Build history of the part. All positions in model axes, mm. A direction names the side the tool comes from. Give positions to 0.01 mm unless a question says otherwise; leave off trailing zeros. Order: outer loops, then holes, each group sorted by start corner. A loop starts at its lowest first (then second) coordinate and runs counter-clockwise, first axis right, second up. Notation, with made-up numbers: (-10, 42) - (12, 42) arc R13 ccw to (12, 58) - close; hole circle Ø1 at (37, 29.5). An arc over 180 degrees is marked (long way). Use a Markdown table: item, result.
Autodesk Inventor part; units mm, degrees
ref_plane "YZ Plane" through (0, 0, 0) normal (1, 0, 0) x (0, 1, 0)
ref_plane "XZ Plane" through (0, 0, 0) normal (0, 1, 0) x (-1, 0, 0)
ref_plane "XY Plane" through (0, 0, 0) normal (0, 0, 1) x (1, 0, 0)
sketch "Boceto1" plane through (0, 0, 0) normal (0, 1, 0) x (-1, 0, 0)
  circle A0 centre (0, 0) radius 10.2
  circle A1 centre (0, 0) radius 12.2
  dimension "d0" = 20.4
  dimension "d1" = 2
extrude "Extrusión1" add sketch "Boceto1" along normal blind 2
sketch "Boceto2" plane through (0, 2, 0) normal (0, 1, 0) x (1, 0, 0)
  circle A0 centre (0, 0) radius 12.2
  circle A1 centre (0, 0) radius 10.2
  circle A2 centre (0, 0) radius 2.25
  dimension "d4" = 4.5
extrude "Extrusión2" add sketch "Boceto2" along normal blind 4 contours A0 | A1
sketch "Boceto3" plane through (0, 6, 0) normal (0, 1, 0) x (1, 0, 0)
  circle A0 centre (0, 0) radius 5
  dimension "d7" = 10
extrude "Extrusión3" cut sketch "Boceto3" against normal blind 2
properties part number "springsupport"
1) Wall check: line 1 (X direction, y = 5.4, z = 0); line 2 (Z direction, x = 0, y = 3.25). Give the ranges that are in metal, low to high. Write a range as from..to.
Computed:
| item | result |
|---|---|
| line 1 | x = -12.2..-5, 5..12.2 |
| line 2 | z = -12.2..-2.25, 2.25..12.2 |
2) Slice it at B-B (z = -1). Write the cut outline in (x, y), and give its area (3 significant figures).
Computed:
| item | result |
|---|---|
| outline | (-12.16, 0) - (-10.15, 0) - (-10.15, 2) - (-2.02, 2) - (-2.02, 4) - (-4.9, 4) - (-4.9, 6) - (-12.16, 6) - close; (2.02, 2) - (10.15, 2) - (10.15, 0) - (12.16, 0) - (12.16, 6) - (4.9, 6) - (4.9, 4) - (2.02, 4) - close |
| area | 77.6 mm² |
3) Tool access for faces 1 (the flat face through (-0.1, 2, -2.4)), 2 (the flat face through (2.2, 4, 1)), 3 (the flat face through (3, 0, -10)): list every direction of +Z, -Z, +X, -X, +Y, -Y with a clear straight run to the whole face (end or side of a thin tool).
Computed:
| item | result |
|---|---|
| face 1 | -Y |
| face 2 | +Y |
| face 3 | +Z, -Z, +X, -X, -Y |
4) Pin check, flat tips, straight feed: P1, Ø1, axis at x = -10, y = 3, coming from the -Z side; P2, Ø7, axis at x = 0, z = 0, coming from the -Y side; P3, Ø3, axis at x = 2, z = 2.5, coming from the +Y side. Stop position of each tip, or through.
Computed:
| item | result |
|---|---|
| P1 | stops at z = -7.65 |
| P2 | stops at y = 2 |
| P3 | stops at y = 4 |
5) Slice it at C-C (y = 5.1). Write the cut outline in (x, z), and give its area (3 significant figures).
Computed:
| item | result |
|---|---|
| outline | circle Ø24.4 at (0, 0); hole circle Ø10 at (0, 0) |
| area | 389 mm² |
6) Two-plate mould, pull along Z, no slides. Class faces 4 (the cylindrical face through (-1.08, 5.01, 4.88)), 5 (the cylindrical face through (0.804, 2.958, 12.173)), 6 (the flat face through (5.3, 6, -0.2)), 7 (the cylindrical face through (-4.707, 0.986, 9.049)): +Z half, -Z half, draft (parallel to the pull), parting line (faces both ways), or undercut.
Computed:
| item | result |
|---|---|
| face 4 | undercut |
| face 5 | parting line |
| face 6 | draft |
| face 7 | undercut |
7) Slice it at D-D (z = -8.75). Write the cut outline in (x, y).
Computed:
| item | result |
|---|---|
| outline | (-8.5, 0) - (-5.24, 0) - (-5.24, 2) - (5.24, 2) - (5.24, 0) - (8.5, 0) - (8.5, 6) - (-8.5, 6) - close |
